Part model, mm, in its own coordinate system. A direction names the side the tool comes from. Round coordinates to 2 decimals unless told otherwise and drop trailing zeros. Write each loop counter-clockwise with the first axis right and the second up, starting at its lowest first coordinate (ties: lowest second). Pieces come first, ordered by that corner, then holes. Notation, with made-up numbers: (-1.75, 48.25) -> (36.25, 48.25) arc R23 cw to (36.25, 78.25) -> close; hole circle Ø10 at (67.5, 69.25). An arc over 180 degrees is marked (long way). Return JSON: item names as keys, results as strings. Group by question number.
(1) Saw through at B-B (z = -1). List the corners of the cut face in (x, y).
(2) Saw through at C-C (y = 1.45). List the corners of the cut face in (x, z), plus the area to 3 significant figures.
(3) Mould opens along X. For faces 1 (the cylindrical face through (-4.1, -1.5, 0.1)), 2 (the cylindrical face through (54.8, 0.5, 0.1)), 3 (the flat face through (19, 0, -6)) say: +X half, -X half, draft (parallel to the pull), parting line (faces both ways), or undercut.
(4) Tool access for faces 4 (the flat face through (13, 1, 1.5)), 5 (the flat face through (9.54, -1.48, -3.35)), 6 (the cylindrical face through (-6, 0, 0)): list every direction of +Z, -Z, +X, -X, +Y, -Y with a clear straight run to the whole face (end or side of a thin tool).
(5) Saw through at D-D (z = 4.75). List the corners of the cut face in (x, y).
(6) Drop flat-ended pins along their axis: pin 1 Ø6 at (x, z) = (40, 2.5) entering from -Y; pin 2 Ø1 at (y, z) = (-1.5, -0.5) entering from -X. Give the stop position or say it passes through.
(7) Drill centre lines: L1, parallel to Z at x = 33, y = 0.05; L2, parallel to Y at x = 4, z = 2.25; L3, parallel to X at y = -1.75, z = 0.5. Where is each one in solid material? Low to high. Write a range as from..to.
(8) Saw through at A-A (y = -1.7). List the corners of the cut face in (x, z), plus the area to 3 significant figures.
from build123d import *

# Parameters (mm, degrees)
EXTRUDE_1_DEPTH     = 3
EXTRUDE_START       = 2
SKETCH_1_4_R        = 2.35
EXTRUDE_2_DEPTH     = 2
EXTRUDE_3_DEPTH     = 3
CUT_EXTRUDE_1_DEPTH = 10


with BuildPart() as part:
    # Sketch 1 → Extrude 1 (new body)
    with BuildSketch(Plane(origin=(0, 0, 0), x_dir=(1, 0, 0), z_dir=(0, 1, 0))):
        with BuildLine():
            ThreePointArc((18.8, -6), (24.8, 0), (18.8, 6))
            Line((18.8, 6), (0, 6))
            ThreePointArc((0, 6), (-6, 0), (0, -6))
            Line((0, -6), (18.8, -6))
        make_face()
        with BuildLine():
            ThreePointArc((0.32712766, -4.086928858), (-4.1, 0), (0.32712766, 4.086928858))
            Line((0.32712766, 4.086928858), (19.007446809, 2.591710983))
            ThreePointArc((19.007446809, 2.591710983), (21.4, 0), (19.007446809, -2.591710983))
            Line((19.007446809, -2.591710983), (0.32712766, -4.086928858))
        make_face(mode=Mode.SUBTRACT)
    extrude(amount=-EXTRUDE_1_DEPTH)

    # Sketch 1_4 → Extrude 2 (add)
    with BuildSketch(Plane(origin=(0, 0, 0), x_dir=(1, 0, 0), z_dir=(0, 1, 0)).offset(EXTRUDE_START)):
        with BuildLine():
            ThreePointArc((18.8, -6), (24.8, 0), (18.8, 6))
            Line((18.8, 6), (0, 6))
            ThreePointArc((0, 6), (-6, 0), (0, -6))
            Line((0, -6), (18.8, -6))
        make_face()
        with Locations(Location((0, 0, 0), (0, 0, 270))):
            Circle(SKETCH_1_4_R, mode=Mode.SUBTRACT)
    extrude(amount=-EXTRUDE_2_DEPTH)

    # Sketch 2 → Extrude 3 (add)
    with BuildSketch(Plane(origin=(0, 2, 0), x_dir=(1, 0, 0), z_dir=(0, 1, 0))):
        with BuildLine():
            ThreePointArc((48.8, -6), (54.8, 0), (48.8, 6))
            Line((48.8, 6), (18.8, 6))
            ThreePointArc((18.8, 6), (24.8, 0), (18.8, -6))
            Line((18.8, -6), (48.8, -6))
        make_face()
        with BuildLine():
            ThreePointArc((48.8, 1.75), (50.55, 0), (48.8, -1.75))
            Line((48.8, -1.75), (28.8, -1.75))
            ThreePointArc((28.8, -1.75), (27.05, 0), (28.8, 1.75))
            Line((28.8, 1.75), (48.8, 1.75))
        make_face(mode=Mode.SUBTRACT)
    extrude(amount=-EXTRUDE_3_DEPTH)

    # Sketch 2_3 → Cut-Extrude 1 (cut)
    with BuildSketch(Plane(origin=(0, 2, 0), x_dir=(1, 0, 0), z_dir=(0, 1, 0))):
        with BuildLine():
            ThreePointArc((6.8, -1.5), (7.860660172, -1.060660172), (8.3, 0))
            Line((8.3, 0), (5.3, 0))
            ThreePointArc((5.3, 0), (5.739339828, -1.060660172), (6.8, -1.5))
        make_face()
        with BuildLine():
            Line((5.3, 0), (8.3, 0))
            ThreePointArc((8.3, 0), (7.860660172, 1.060660172), (6.8, 1.5))
            ThreePointArc((6.8, 1.5), (5.739339828, 1.060660172), (5.3, 0))
        make_face()
        with BuildLine():
            Line((8.3, 0), (17.3, 0))
            ThreePointArc((17.3, 0), (17.739339828, 1.060660172), (18.8, 1.5))
            Line((18.8, 1.5), (6.8, 1.5))
            ThreePointArc((6.8, 1.5), (7.860660172, 1.060660172), (8.3, 0))
        make_face()
        with BuildLine():
            ThreePointArc((18.8, -1.5), (17.739339828, -1.060660172), (17.3, 0))
            Line((17.3, 0), (8.3, 0))
            ThreePointArc((8.3, 0), (7.860660172, -1.060660172), (6.8, -1.5))
            Line((6.8, -1.5), (18.8, -1.5))
        make_face()
        with BuildLine():
            ThreePointArc((18.8, -1.5), (19.860660172, -1.060660172), (20.3, 0))
            Line((20.3, 0), (17.3, 0))
            ThreePointArc((17.3, 0), (17.739339828, -1.060660172), (18.8, -1.5))
        make_face()
        with BuildLine():
            Line((17.3, 0), (20.3, 0))
            ThreePointArc((20.3, 0), (19.860660172, 1.060660172), (18.8, 1.5))
            ThreePointArc((18.8, 1.5), (17.739339828, 1.060660172), (17.3, 0))
        make_face()
    extrude(amount=-CUT_EXTRUDE_1_DEPTH, mode=Mode.SUBTRACT)


solid = part.part
Computed values:
{
 "1": {"outline": "(-5.92, -3) -> (-3.98, -3) -> (-3.98, 0) -> (-2.13, 0) -> (-2.13, 2) -> (-5.92, 2) -> close; (2.13, 0) -> (5.68, 0) -> (5.68, 2) -> (2.13, 2) -> close; (19.92, 0) -> (21.2, 0) -> (21.2, -3) -> (24.72, -3) -> (24.72, -1) -> (27.36, -1) -> (27.36, 2) -> (19.92, 2) -> close; (50.24, -1) -> (54.72, -1) -> (54.72, 2) -> (50.24, 2) -> close"},
 "2": {"outline": "(0, -6) -> (48.8, -6) arc R6 ccw to (48.8, 6) -> (0, 6) arc R6 ccw to start; hole circle Ø4.7 at (0, 0); hole (6.8, -1.5) -> (18.8, -1.5) arc R1.5 ccw to (18.8, 1.5) -> (6.8, 1.5) arc R1.5 ccw to start; hole (28.8, -1.75) -> (48.8, -1.75) arc R1.75 ccw to (48.8, 1.75) -> (28.8, 1.75) arc R1.75 ccw to start", "area": "559 mm2"},
 "3": {"face 1": "undercut", "face 2": "+X half", "face 3": "draft"},
 "4": {"face 4": "+Y, -Y", "face 5": "-Y", "face 6": "-X, +Y, -Y"},
 "5": {"outline": "(-3.67, -3) -> (22.47, -3) -> (22.47, -1) -> (52.47, -1) -> (52.47, 2) -> (-3.67, 2) -> close"},
 "6": {"pin 1": "y = -1", "pin 2": "x = -6"},
 "7": {"L1": "-6..-1.75, 1.75..6", "L2": "0..2", "L3": "-5.98..-4.07, 21.35..24.78"},
 "8": {"outline": "(0, -6) -> (18.8, -6) arc R6 ccw to (18.8, 6) -> (0, 6) arc R6 ccw to start; hole (0.33, -4.09) -> (19.01, -2.59) arc R2.6 ccw to (19.01, 2.59) -> (0.33, 4.09) arc R4.1 ccw (long way) to start", "area": "175 mm2"}
}
